Work out the finished part from the listing and answer in its coordinate system (mm). Round coordinates to 2 decimals unless told otherwise and drop trailing zeros. Loops run counter-clockwise (first coordinate to the right, second up) from the corner with the lowest first, then second, coordinate; pieces in that order, holes last.
```python
from build123d import *

# Parameters (mm, degrees)
F0_W     = 65
F0_H     = 6
F0_W_2   = 130
F1_DEPTH = 6


with BuildPart() as f1:
    # F0 (on Top) → F1 (new body)
    with BuildSketch(Plane.XY):
        with BuildLine():
            Line((-172.914558, 23.37498), (-183.537395, 68.384158))
            ThreePointArc((-183.537395, 68.384158), (-188.503299, 75.22998), (-196.863512, 76.507601))
            ThreePointArc((-196.863512, 76.507601), (-211.276495, 71.361563), (-223.12419, 61.674048))
            Line((-223.12419, 61.674048), (-243.158294, -6.624031))
            Line((-243.158294, -6.624031), (286.841706, -6.624031))
            Line((286.841706, -6.624031), (286.841706, 14.214297))
            ThreePointArc((286.841706, 14.214297), (228.846641, 19.825852), (170.610839, 21.698951))
            Line((170.610839, 21.698951), (32.24461, 21.698951))
            Line((32.24461, 21.698951), (31.802109, 25.625584))
            ThreePointArc((31.802109, 25.625584), (26.712862, 35.070635), (16.50378, 38.369733))
            ThreePointArc((16.50378, 38.369733), (-6.900195, 38.178785), (-30.239211, 36.425835))
            ThreePointArc((-30.239211, 36.425835), (-96.427228, 28.654331), (-161.946659, 16.470163))
            ThreePointArc((-161.946659, 16.470163), (-168.84401, 17.677466), (-172.914558, 23.37498))
        make_face()
        with Locations((-158.532006, 2.002824)):
            Rectangle(F0_W, F0_H, mode=Mode.SUBTRACT)
        with BuildLine():
            Line((286.841706, -6.624031), (-243.158294, -6.624031))
            ThreePointArc((-243.158294, -6.624031), (-241.41439, -16.025181), (-232.804301, -20.183209))
            Line((-232.804301, -20.183209), (-194.829215, -26.364981))
            ThreePointArc((-194.829215, -26.364981), (-82.594257, -43.652901), (30.72672, -50.995535))
            Line((30.72672, -50.995535), (158.609955, -53.635519))
            ThreePointArc((158.609955, -53.635519), (216.073845, -56.007438), (273.170183, -49.09854))
            ThreePointArc((273.170183, -49.09854), (279.335818, -41.281654), (281.455098, -31.553993))
            Line((281.455098, -31.553993), (281.330585, -21.315108))
            ThreePointArc((281.330585, -21.315108), (282.952438, -17.537773), (286.841706, -16.206507))
            Line((286.841706, -16.206507), (286.841706, -6.624031))
        make_face()
        with Locations((100.650969, -32.257092)):
            Rectangle(F0_W_2, F0_H, mode=Mode.SUBTRACT)
    extrude(amount=F1_DEPTH)


solid = f1.part
```
1. Determine the mould class of faces 1 (the face through (-178.15, 45.56, 2.96)), 2 (the face through (-233, 28, 3)), 3 (the face through (-95.505, 28.794, 2.958)), 4 (the face through (279.275, -41.409, 2.958)) for opening direction X: +X half, -X half, draft (parallel to the pull), parting line (faces both ways), or undercut.
Answer key:
face 1: undercut
face 2: -X half
face 3: undercut
face 4: +X half
2. Consider probe 1 along Y at (x, z) = (83, 3.8); probe 2 along Y at (x, z) = (-169.5, 1.65); probe 3 along Y at (x, z) = (179, 3.2). Determine where each line is inside the solid, lowest interval first.
Answer key:
probe 1: y = -52.07 to -35.26, -29.26 to 21.7
probe 2: y = -31.15 to -1, 5 to 18.13
probe 3: y = -55.54 to 21.66
3. Find section B-B (z = 4). Write down the section's boundary in (x, y), then the cut area to 3 significant figures.
Answer key:
outline: (-243.16, -6.62) arc R10.58 ccw to (-232.8, -20.18) - (-194.83, -26.36) arc R1288.99 ccw to (30.73, -51) - (158.61, -53.64) arc R356.13 ccw to (273.17, -49.1) arc R22.15 ccw to (281.46, -31.55) - (281.33, -21.32) arc R5.07 cw to (286.84, -16.21) - (286.84, 14.21) arc R906.23 ccw to (170.61, 21.7) - (32.24, 21.7) - (31.8, 25.63) arc R14.39 ccw to (16.5, 38.37) arc R350.39 ccw to (-30.24, 36.43) arc R995.12 ccw to (-161.95, 16.47) arc R9.24 cw to (-172.91, 23.37) - (-183.54, 68.38) arc R10.97 ccw to (-196.86, 76.51) arc R44.9 ccw to (-223.12, 61.67) - close; hole (-191.03, -1) - (-126.03, -1) - (-126.03, 5) - (-191.03, 5) - close; hole (35.65, -35.26) - (165.65, -35.26) - (165.65, -29.26) - (35.65, -29.26) - close
area: 38,100 mm2
4. Find section C-C (y = 49). Write down the section's boundary in (x, z), then the cut area to 3 significant figures.
Answer key:
outline: (-226.84, 0) - (-178.96, 0) - (-178.96, 6) - (-226.84, 6) - close
area: 287 mm2
5. Find section D-D (x = 192). Write down the section's boundary in (y, z).
Answer key:
outline: (-56.15, 0) - (21.45, 0) - (21.45, 6) - (-56.15, 6) - close
6. Find section A-A (x = 83.5). Write down the section's boundary in (y, z).
Answer key:
outline: (-52.08, 0) - (-35.26, 0) - (-35.26, 6) - (-52.08, 6) - close; (-29.26, 0) - (21.7, 0) - (21.7, 6) - (-29.26, 6) - close
7. Given pin 1 (1 mm diameter, centred on y = -7, z = 5, fed in from -X); pin 2 (3 mm diameter, centred on x = -167, z = 2.5, fed in from +Y); pin 3 (3 mm diameter, centred on x = 99.5, z = 2, fed in from +Y), each flat-ended and moving along its own axis, determine where each tip first touches the part or whether it passes through.
Answer key:
pin 1: stops at x = -243.38
pin 2: stops at y = 17.47
pin 3: stops at y = 21.7
